Geometry check sheet. Reference: the model listing, model coordinates, mm. Face numbers are marked on the shaded views. A direction names the side the tool comes from. Round coordinates to 2 decimals unless told otherwise and drop trailing zeros. Loops run counter-clockwise (first coordinate to the right, second up) from the corner with the lowest first, then second, coordinate; pieces in that order, holes last. Notation, with made-up numbers: M 82,-22.75 L 137,-22.75 A10 cw 137,-15.75 Z; hole C 67,3 d11. An arc over 180 degrees is marked long. Use one line per item in the form item = value. Start each with the question number.
1. Cross-section at B-B (y = 1.25). Record the boundary of the cut face in (x, z), then the cut area to 3 significant figures.
2. Set-up check for the marked faces 4 and 5: record each of +Z, -Z, +X, -X, +Y, -Y from which the full face is reachable in a straight line by a thin tool's end or side.
3. Material ranges on line 1 (X direction, y = 10.25, z = 0); line 2 (Z direction, x = 10, y = 5); line 3 (X direction, y = 2.25, z = 9.5), recorded low to high.
4. Go/stop test with flat-tipped pins: pin 1 (10 mm diameter, centred on x = 1, z = -2, fed in from +Y); pin 2 (3 mm diameter, centred on x = -7.5, y = 7, fed in from +Z); pin 3 (10 mm diameter, centred on x = -15.5, y = 9, fed in from -Z); pin 4 (21 mm diameter, centred on x = -9.5, z = -2.5, fed in from +Y). Record where each tip stops, or that it passes through.
5. Draft check along Z on the marked faces 1, 2 and 3. Enter one of: pulls with the +Z half, pulls with the -Z half, needs draft (parallel to the pull), parting line crosses it, or undercut.
6. Cross-section at A-A (x = 0). Record the boundary of the cut face in (y, z), then the cut area to 3 significant figures.
7. Cross-section at C-C (y = -3.25). Record the boundary of the cut face in (x, z).
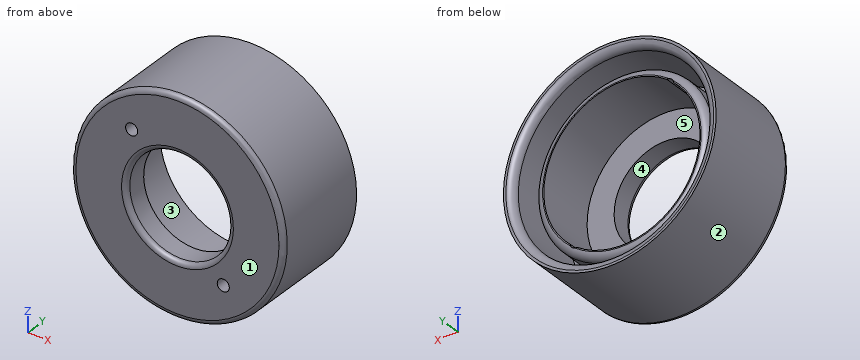
```python
from build123d import *

# Parameters (mm, degrees)
CROQUIS1_R              = 22.05
CROQUIS1_R_2            = 20.05
SALIENTE_EXTRUIR1_DEPTH = 16
CROQUIS1_4_R            = 17.95
CROQUIS1_4_R_2          = 16.2
SALIENTE_EXTRUIR2_DEPTH = 12.5
SALIENTE_EXTRUIR4_START = -5
CROQUIS1_6_R            = 22.05
CROQUIS1_6_R_2          = 20.05
CROQUIS1_6_R_3          = 17.95
CROQUIS1_6_R_4          = 16.2
SALIENTE_EXTRUIR4_DEPTH = 5
CORTAR_EXTRUIR1_REACH   = 39.595
CROQUIS4_R              = 10.6
CROQUIS4_R_2            = 1.25
REDONDEO1_R             = 1
REDONDEO2_R             = 1.5
REDONDEO3_R             = 1


with BuildPart() as part:
    # Croquis1 → Saliente-Extruir1 (new body)
    with BuildSketch(Plane(origin=(0, 0, 0), x_dir=(1, 0, 0), z_dir=(0, 1, 0))):
        with Locations(Location((0, 0, 0), (0, 0, 270))):
            Circle(CROQUIS1_R)
        with Locations(Location((0, 0, 0), (0, 0, 270))):
            Circle(CROQUIS1_R_2, mode=Mode.SUBTRACT)
    extrude(amount=SALIENTE_EXTRUIR1_DEPTH)



with BuildPart() as body_2:
    # Croquis1<4> → Saliente-Extruir2 (new body)
    with BuildSketch(Plane(origin=(0, 0, 0), x_dir=(1, 0, 0), z_dir=(0, 1, 0))):
        with Locations(Location((0, 0, 0), (0, 0, 270))):
            Circle(CROQUIS1_4_R)
        with Locations(Location((0, 0, 0), (0, 0, 270))):
            Circle(CROQUIS1_4_R_2, mode=Mode.SUBTRACT)
    extrude(amount=SALIENTE_EXTRUIR2_DEPTH)


with BuildPart() as part_1:
    add(part.part)

    add(body_2.part)  # Saliente-Extruir4 merges body 2
    # Croquis1<6> → Saliente-Extruir4 (add)
    # profile 1 of 4: a face of its own
    with BuildSketch(Plane(origin=(0, 0, 0), x_dir=(1, 0, 0), z_dir=(0, 1, 0)).offset(SALIENTE_EXTRUIR4_START)):
        with Locations(Location((0, 0, 0), (0, 0, 270))):
            Circle(CROQUIS1_6_R)
        with Locations(Location((0, 0, 0), (0, 0, 270))):
            Circle(CROQUIS1_6_R_2, mode=Mode.SUBTRACT)
    # profile 2 of 4: a face of its own
    with BuildSketch(Plane(origin=(0, 0, 0), x_dir=(1, 0, 0), z_dir=(0, 1, 0)).offset(SALIENTE_EXTRUIR4_START)):
        with Locations(Location((0, 0, 0), (0, 0, 270))):
            Circle(CROQUIS1_6_R_2)
        with Locations(Location((0, 0, 0), (0, 0, 270))):
            Circle(CROQUIS1_6_R_3, mode=Mode.SUBTRACT)
    # profile 3 of 4: a face of its own
    with BuildSketch(Plane(origin=(0, 0, 0), x_dir=(1, 0, 0), z_dir=(0, 1, 0)).offset(SALIENTE_EXTRUIR4_START)):
        with Locations(Location((0, 0, 0), (0, 0, 270))):
            Circle(CROQUIS1_6_R_3)
        with Locations(Location((0, 0, 0), (0, 0, 270))):
            Circle(CROQUIS1_6_R_4, mode=Mode.SUBTRACT)
    # profile 4 of 4: a face of its own
    with BuildSketch(Plane(origin=(0, 0, 0), x_dir=(1, 0, 0), z_dir=(0, 1, 0)).offset(SALIENTE_EXTRUIR4_START)):
        with Locations(Location((0, 0, 0), (0, 0, 270))):
            Circle(CROQUIS1_6_R_4)
    extrude(amount=SALIENTE_EXTRUIR4_DEPTH)

    # Croquis4 → Cortar-Extruir1 (cut, up to next)
    with BuildSketch(Plane.XZ.offset(5), mode=Mode.PRIVATE) as cortar_extruir1_sk1:
        with Locations(Location((0, 0, 0), (0, 0, 270))):
            Circle(CROQUIS4_R)
    cortar_extruir1_tool1 = extrude(cortar_extruir1_sk1.sketch, amount=-CORTAR_EXTRUIR1_REACH, mode=Mode.PRIVATE) & part_1.part
    # Croquis4 → Cortar-Extruir1 (cut, up to next)
    with BuildSketch(Plane.XZ.offset(5), mode=Mode.PRIVATE) as cortar_extruir1_sk2:
        with Locations(Location((-9.5, 12, 0), (0, 0, 270))):
            Circle(CROQUIS4_R_2)
    cortar_extruir1_tool2 = extrude(cortar_extruir1_sk2.sketch, amount=-CORTAR_EXTRUIR1_REACH, mode=Mode.PRIVATE) & part_1.part
    # Croquis4 → Cortar-Extruir1 (cut, up to next)
    with BuildSketch(Plane.XZ.offset(5), mode=Mode.PRIVATE) as cortar_extruir1_sk3:
        with Locations(Location((9.5, -12, 0), (0, 0, 270))):
            Circle(CROQUIS4_R_2)
    cortar_extruir1_tool3 = extrude(cortar_extruir1_sk3.sketch, amount=-CORTAR_EXTRUIR1_REACH, mode=Mode.PRIVATE) & part_1.part
    add(cortar_extruir1_tool1.solids().sort_by_distance((0, -5, 0))[0], mode=Mode.SUBTRACT)
    add(cortar_extruir1_tool2.solids().sort_by_distance((-9.5, -5, 12))[0], mode=Mode.SUBTRACT)
    add(cortar_extruir1_tool3.solids().sort_by_distance((9.5, -5, -12))[0], mode=Mode.SUBTRACT)

    # Redondeo1
    redondeo1_edges = [part_1.edges().sort_by_distance(p)[0] for p in [
        (0, -5, 10.6),
    ]]
    fillet(redondeo1_edges, radius=REDONDEO1_R)

    # Redondeo2
    # the kernel refuses this fillet: 1.5 mm, written as the material it takes off along each edge
    with BuildSketch(Plane(origin=(0, 12.5, 0), x_dir=(0, 0, 1), z_dir=(-1, 0, 0))) as redondeo2_piece_1:
        with BuildLine():
            CenterArc((17.95 - REDONDEO2_R, -REDONDEO2_R), REDONDEO2_R, 0, 90)
            Line((17.95, -REDONDEO2_R), (17.95, 0))
            Line((17.95, 0), (17.95 - REDONDEO2_R, 0))
        make_face()
    revolve(axis=Axis((0, 12.5, 0), (0, 1, 0)), mode=Mode.SUBTRACT)
    with BuildSketch(Plane(origin=(0, 16, 0), x_dir=(0, 0, 1), z_dir=(-1, 0, 0))) as redondeo2_piece_2:
        with BuildLine():
            CenterArc((20.05 + REDONDEO2_R, -REDONDEO2_R), REDONDEO2_R, 90, 90)
            Line((20.05, -REDONDEO2_R), (20.05, 0))
            Line((20.05, 0), (20.05 + REDONDEO2_R, 0))
        make_face()
    revolve(axis=Axis((0, 16, 0), (0, 1, 0)), mode=Mode.SUBTRACT)

    # Redondeo3
    redondeo3_edges = [part_1.edges().sort_by_distance(p)[0] for p in [
        (0, -5, -22.05),
    ]]
    fillet(redondeo3_edges, radius=REDONDEO3_R)


solid = part_1.part
```
Reported:
q1.outline = C 0,0 d44.1; C 0,0 d35.9; hole C 0,0 d40.1; hole M -10.74,12.12 A16.2 ccw 9.34,-13.24 A1.25 ccw 10.74,-12.12 A16.2 ccw -9.34,13.24 A1.25 ccw Z
q1.area = 451 mm²
q2.face_4 = +Y, -Y
q2.face_5 = +Y
q3.line_1 = -22.05 to -20.05, -17.95 to -16.2, 16.2 to 17.95, 20.05 to 22.05
q3.line_2 = -19.65 to -17.38, -14.91 to -13.15, 12.75 to 14.91, 17.38 to 19.65
q3.line_3 = -19.9 to -17.66, -15.23 to -13.12, 13.12 to 15.23, 17.66 to 19.9
q4.pin_1 = through
q4.pin_2 = 21.22
q4.pin_3 = -19.39
q4.pin_4 = 15.36
q5.face_1 = needs draft
q5.face_2 = parting line crosses it
q5.face_3 = undercut
q6.outline = M -5,-21.05 A1 ccw -4,-22.05 L 16,-22.05 L 16,-21.55 A1.5 ccw 14.5,-20.05 L 0,-20.05 L 0,-17.95 L 11,-17.95 A1.5 ccw 12.5,-16.45 L 12.5,-16.2 L 0,-16.2 L 0,-10.6 L -4,-10.6 A1 ccw -5,-11.6 Z; M -5,11.6 A1 ccw -4,10.6 L 0,10.6 L 0,16.2 L 12.5,16.2 L 12.5,16.45 A1.5 ccw 11,17.95 L 0,17.95 L 0,20.05 L 14.5,20.05 A1.5 ccw 16,21.55 L 16,22.05 L -4,22.05 A1 ccw -5,21.05 Z
q6.area = 219 mm²
q7.outline = C 0,0 d44.1; hole C -9.5,12 d2.5; hole C 0,0 d21.2; hole C 9.5,-12 d2.5
